```python
from build123d import *

# Parameters (mm, degrees)
CONTOURS_R              = 0.996805003
CONTOURS_R_2            = 0.884493699
CONTOURS_R_3            = 0.969462683
CONTOURS_R_4            = 0.92016771
BOSS_EXTRU_1_DEPTH      = 3
ENL_V_MAT_EXTRU_3_DEPTH = 0.5
ESQUISSE6_R             = 0.92016771
ESQUISSE6_R_2           = 0.969462683
BOSS_EXTRU_2_DEPTH      = 2.5
ESQUISSE7_W             = 65.577757284
ESQUISSE7_H             = 1.135573616
ESQUISSE7_W_2           = 65.714172828
ESQUISSE7_H_2           = 1.121624069
ESQUISSE7_H_3           = 1.147393865
BOSS_EXTRU_3_DEPTH      = 1
ESQUISSE8_W             = 63.110312129
ESQUISSE8_H             = 6.788838012
ESQUISSE8_H_2           = 6.737736788
ESQUISSE8_H_3           = 6.757335266
BOSS_EXTRU_4_DEPTH      = 1.3
ESQUISSE12_W            = 0.779629517
ESQUISSE12_H            = 6.41876269
ESQUISSE12_W_2          = 0.785524209
BOSS_EXTRU_6_DEPTH      = 3
CHANFREIN1_SIZE         = 2
CHANFREIN2_SIZE         = 2


with BuildPart() as part:
    # Contours → Boss.-Extru.1 (new body)
    with BuildSketch(Plane.XY):
        with BuildLine():
            Line((-13.53709508, 8.689037277), (49.427183341, 8.689037277))
            Line((49.427183341, 8.689037277), (49.427183341, -15.576035195))
            Line((49.427183341, -15.576035195), (49.427183341, -16.167014971))
            Line((49.427183341, -16.167014971), (48.103014513, -17.491183799))
            Line((48.103014513, -17.491183799), (47.222080517, -17.491183799))
            Line((47.222080517, -17.491183799), (46.905484209, -19.797319309))
            Line((46.905484209, -19.797319309), (46.377823694, -21.422513692))
            Line((46.377823694, -21.422513692), (45.61180941, -21.813030779))
            Line((45.61180941, -21.813030779), (43.444031236, -22.119025571))
            Line((43.444031236, -22.119025571), (40.627206664, -22.516637126))
            Line((40.627206664, -22.516637126), (36.607696599, -23.084014896))
            Line((36.607696599, -23.084014896), (33.650652093, -23.364304384))
            Line((33.650652093, -23.364304384), (30.65446793, -25.457235805))
            Line((30.65446793, -25.457235805), (5.129220902, -25.457235805))
            Line((5.129220902, -25.457235805), (3.210082619, -27.376374088))
            Line((3.210082619, -27.376374088), (3.086468117, -27.469210212))
            Line((3.086468117, -27.469210212), (1.882461508, -27.469210212))
            Line((1.882461508, -27.469210212), (1.368391271, -27.144534273))
            Line((1.368391271, -27.144534273), (1.152232663, -27.306872243))
            Line((1.152232663, -27.306872243), (0.691983064, -27.306872243))
            Line((0.691983064, -27.306872243), (-0.167684887, -26.763924063))
            Line((-0.167684887, -26.763924063), (-0.49849538, -26.416804947))
            Line((-0.49849538, -26.416804947), (-2.55477633, -25.588795397))
            Line((-2.55477633, -25.588795397), (-2.653579321, -25.457235805))
            Line((-2.653579321, -25.457235805), (-2.653579321, -23.084014896))
            Line((-2.653579321, -23.084014896), (-3.036044011, -22.701550207))
            Line((-3.036044011, -22.701550207), (-9.780970444, -21.775577383))
            Line((-9.780970444, -21.775577383), (-10.358479282, -21.543029961))
            Line((-10.358479282, -21.543029961), (-10.639580473, -21.168734027))
            Line((-10.639580473, -21.168734027), (-10.823901747, -20.609916501))
            Line((-10.823901747, -20.609916501), (-10.916488176, -19.954000633))
            Line((-10.916488176, -19.954000633), (-11.060291782, -18.935243689))
            Line((-11.060291782, -18.935243689), (-11.184195314, -17.628065669))
            ThreePointArc((-11.184195314, -17.628065669), (-11.230466887, -17.54072814), (-11.324942788, -17.511690124))
            Line((-11.324942788, -17.511690124), (-12.261208369, -17.442093435))
            Line((-12.261208369, -17.442093435), (-12.746327303, -16.956974502))
            Line((-12.746327303, -16.956974502), (-13.411955607, -16.291346198))
            Line((-13.411955607, -16.291346198), (-13.59975919, -16.167014971))
            Line((-13.59975919, -16.167014971), (-13.683128788, -15.023442521))
            Line((-13.683128788, -15.023442521), (-13.683128788, 8.689037277))
            Line((-13.683128788, 8.689037277), (-13.53709508, 8.689037277))
        make_face()
        with Locations((45.140288013, -20.300965513)):
            Circle(CONTOURS_R, mode=Mode.SUBTRACT)
        with Locations((-9.263810849, -20.300965513)):
            Circle(CONTOURS_R_2, mode=Mode.SUBTRACT)
        with Locations((-7.107072771, 0.361135268)):
            Circle(CONTOURS_R_3, mode=Mode.SUBTRACT)
        with Locations((17.950565341, 0.361135268)):
            Circle(CONTOURS_R_4, mode=Mode.SUBTRACT)
        with Locations((42.975492251, 0.361135268)):
            Circle(CONTOURS_R_4, mode=Mode.SUBTRACT)
    extrude(amount=BOSS_EXTRU_1_DEPTH)

    # Esquisse5 → Enlèv. mat.-Extru.3 (cut)
    with BuildSketch(Plane.XY.offset(3)):
        Polygon((8.181753212, -14.974213956), (15.937864767, -14.974213956), (15.937864767, -15.592047706), (19.619809184, -15.592047706), (19.619809184, -14.974213956), (27.772380941, -14.974213956), (27.772380941, -24.647748669), (27.308611889, -25.457235805), (8.782258705, -25.457235805), (8.181753212, -24.647748669), align=None)
    extrude(amount=-ENL_V_MAT_EXTRU_3_DEPTH, mode=Mode.SUBTRACT)

    # Esquisse6 → Boss.-Extru.2 (add)
    with BuildSketch(Plane.XY):
        with Locations((42.975492251, 0.361135268)):
            Circle(ESQUISSE6_R)
        with Locations((17.950565341, 0.361135268)):
            Circle(ESQUISSE6_R)
        with Locations((-7.107072771, 0.361135268)):
            Circle(ESQUISSE6_R_2)
    extrude(amount=BOSS_EXTRU_2_DEPTH)

    # Esquisse7 → Boss.-Extru.3 (add)
    with BuildSketch(Plane.XY):
        Polygon((-14.80971951, 8.646615937), (50.768037774, 8.635168208), (50.768037774, 7.517857947), (-14.80971951, 7.517857947), align=None)
        with Locations((17.979159132, 0.161233127)):
            Rectangle(ESQUISSE7_W, ESQUISSE7_H)
        with Locations((17.91095136, -7.705102504)):
            Rectangle(ESQUISSE7_W_2, ESQUISSE7_H_2)
        with Locations((17.91095136, -15.596946737)):
            Rectangle(ESQUISSE7_W_2, ESQUISSE7_H_3)
    extrude(amount=-BOSS_EXTRU_3_DEPTH)

    # Esquisse8 → Boss.-Extru.4 (add)
    with BuildSketch(Plane(origin=(0, 0, 0), x_dir=(-1, 0, 0), z_dir=(0, 0, -1))):
        with Locations((-17.872027276, 4.123438941)):
            Rectangle(ESQUISSE8_W, ESQUISSE8_H)
        with Locations((-17.872027276, -3.775422075)):
            Rectangle(ESQUISSE8_W, ESQUISSE8_H_2)
        with Locations((-17.872027276, -11.644582171)):
            Rectangle(ESQUISSE8_W, ESQUISSE8_H_3)
        with BuildLine():
            Line((-39.947601393, -16.170643669), (3.467572619, -16.170643669))
            Line((3.467572619, -16.170643669), (6.662365967, -16.170643669))
            Line((6.662365967, -16.170643669), (2.928932188, -19.904077448))
            ThreePointArc((2.928932188, -19.904077448), (-0.3153013, -22.071804962), (-4.142135624, -22.833009637))
            Line((-4.142135624, -22.833009637), (-28.712150945, -22.833009637))
            ThreePointArc((-28.712150945, -22.833009637), (-32.297105816, -22.168324231), (-35.405487251, -20.262629351))
            Line((-35.405487251, -20.262629351), (-39.947601393, -16.170643669))
        make_face()
    extrude(amount=BOSS_EXTRU_4_DEPTH)

    # Esquisse12 → Boss.-Extru.6 (add)
    with BuildSketch(Plane.XY.offset(3)):
        with Locations((49.037368583, 4.079655932)):
            Rectangle(ESQUISSE12_W, ESQUISSE12_H)
        with Locations((-13.290366684, 4.079655932)):
            Rectangle(ESQUISSE12_W_2, ESQUISSE12_H)
    extrude(amount=BOSS_EXTRU_6_DEPTH)

    # Chanfrein1
    chanfrein1_edges = [part.edges().sort_by_distance(p)[0] for p in [
        (49.037368582, 7.289037277, 6),
        (49.037368582, 0.870274587, 6),
    ]]
    chamfer(chanfrein1_edges, length=CHANFREIN1_SIZE)

    # Chanfrein2
    chanfrein2_edges = [part.edges().sort_by_distance(p)[0] for p in [
        (-13.290366684, 7.289037277, 6),
        (-13.290366684, 0.870274587, 6),
    ]]
    chamfer(chanfrein2_edges, length=CHANFREIN2_SIZE)


solid = part.part
```
The listing builds one solid part. Answer for the finished solid, in the listing's coordinates (mm). A direction names the side the tool comes from. Round coordinates to 2 decimals unless told otherwise and drop trailing zeros. Loops run counter-clockwise (first coordinate to the right, second up) from the corner with the lowest first, then second, coordinate; pieces in that order, holes last. Notation, with made-up numbers: (-22.5, 69) - (12.5, 69) arc R24 cw to (12.5, 95) - close; hole circle Ø3 at (-33.75, -19.75). An arc over 180 degrees is marked (long way). Use one line per item in the form item = value. Start each with the question number.
1. The part is cut by section A-A on y = 3.5. Determine the outline of the cut face in (x, z), then the cut area to 3 significant figures.
2. The part is cut by section B-B on x = 39. Determine the outline of the cut face in (y, z).
3. Consider line 1 (Z direction, x = -9, y = -14); line 2 (X direction, y = -13.5, z = 1.75); line 3 (Y direction, x = 6.5, z = 1.5). Determine where each line is inside the solid, lowest interval first. Write a range as [from, to].
4. A tool of negligible diameter and unlimited length cuts with its end or side. For faces 1 (the face through (18, 0, -1)), 2 (the face through (17.03, 0.4, 2.75)), 3 (the face through (-12.898, 4, 4)), from which of +Z, -Z, +X, -X, +Y, -Y can it reach the whole face along a straight path? Write none if from no direction.
5. The part is cut by section C-C on z = 1.5. Give the number of separate pieces and of enclosed holes in the cut face, then the cut area to 3 significant figures.
6. Given pin 1 Ø0.8 at (x, z) = (50, -0.5) entering from -Y; pin 2 Ø1.1 at (x, z) = (50, -0.5) entering from +Y; pin 3 Ø1 at (x, y) = (17.5, -22.5) entering from +Z, each flat-ended and moving along its own axis, determine where each tip first touches the part or whether it passes through.
7. The part is cut by section D-D on y = -12. Determine the outline of the cut face in (x, z).
8. For a pull along X with two mould halves and no side action, classify faces 4 (the face through (32.249, -22.187, -0.641)), 5 (the face through (44.144, -20.257, 1.479)), 6 (the face through (17, 8.689, 1)) as pulls with the +X half, pulls with the -X half, needs draft (parallel to the pull), parting line crosses it, or undercut.
Geometry check:
q1.outline = (-13.68, -1.3) - (49.43, -1.3) - (49.43, 6) - (48.65, 6) - (48.65, 3) - (-12.9, 3) - (-12.9, 6) - (-13.68, 6) - close
q1.area = 276 mm^2
q2.outline = (-22.75, 0) - (-17.02, 0) - (-17.02, -1.3) - (-16.17, -1.3) - (-16.17, -1) - (-15.02, -1) - (-15.02, -1.3) - (-8.27, -1.3) - (-8.27, -1) - (-7.14, -1) - (-7.14, -1.3) - (-0.41, -1.3) - (-0.41, -1) - (0.73, -1) - (0.73, -1.3) - (7.52, -1.3) - (7.52, -1) - (8.64, -1) - (8.64, 0) - (8.69, 0) - (8.69, 3) - (-22.75, 3) - close
q3.line_1 = [-1.3, 3]
q3.line_2 = [-13.68, 49.43]
q3.line_3 = [-25.46, 8.69]
q4.face_1 = -Z, +X, -X
q4.face_2 = +Z
q4.face_3 = +Z, +Y, -Y
q5.separate_pieces = 1
q5.enclosed_holes = 2
q5.area = 2,050 mm^2
q6.pin_1 = -16.17
q6.pin_2 = 8.64
q6.pin_3 = 2.5
q7.outline = (-13.68, -1.3) - (49.43, -1.3) - (49.43, 3) - (-13.68, 3) - close
q8.face_4 = pulls with the +X half
q8.face_5 = undercut
q8.face_6 = needs draft
